Geometry check sheet. Reference: the model listing, model coordinates, mm. A direction names the side the tool comes from. Give positions to 0.01 mm unless a question says otherwise; leave off trailing zeros. Write each loop counter-clockwise with the first axis right and the second up, starting at its lowest first coordinate (ties: lowest second). Pieces come first, ordered by that corner, then holes. Notation, with made-up numbers: (76, 3) - (127, 3) arc R20 cw to (127, 7) - close; hole circle Ø11 at (57, 67). An arc over 180 degrees is marked (long way). Use a Markdown table: item, result.
```python
from build123d import *

# Parameters (mm, degrees)
SM_BASE_FLANGE_1_DEPTH = 171
SKETCH_5_OUTSIDE_W     = 426.43
SKETCH_5_OUTSIDE_H     = 439.1
SKETCH_5_OUTSIDE_R     = 515
CUT_EXTRUDE_2_DEPTH    = 250.150713085
FILLET_1_R             = 20
SKETCH_9_R             = 3.3
CUT_EXTRUDE_4_DEPTH    = 250.150713236


# Sheet-metal steps are written as plain solids
with BuildPart() as part:
    # Sketch 1 → Базовая кромка1 (new, symmetric)
    with BuildSketch(Plane.XY):
        with BuildLine():
            Line((150, 0), (-146.676192421, 0))
            ThreePointArc((-146.676192421, 0), (-160.818328044, -4.384471872), (-170, -16))
            Line((-170, -16), (-179.329523032, -12.4))
            ThreePointArc((-179.329523032, -12.4), (-166.475182294, 3.861739379), (-146.676192421, 10))
            Line((-146.676192421, 10), (150, 10))
            Line((150, 10), (150, 0))
        make_face()
    extrude(amount=SM_BASE_FLANGE_1_DEPTH, both=True)

    # Эскиз5 outside → Вырез-Вытянуть2 (cut, through all)
    with BuildSketch(Plane(origin=(0, 10, 0), x_dir=(1, 0, 0), z_dir=(0, 1, 0))):
        with Locations((-14.665, 0)):
            Rectangle(SKETCH_5_OUTSIDE_W, SKETCH_5_OUTSIDE_H)
        with Locations((-365, 0)):
            Circle(SKETCH_5_OUTSIDE_R, mode=Mode.SUBTRACT)
    extrude(amount=-CUT_EXTRUDE_2_DEPTH, mode=Mode.SUBTRACT)


with BuildPart() as cut_extrude_2_kept_piece:
    # of the separate pieces the step leaves, the one the design keeps (cut_extrude_2_pieces_kept)
    add(part.part.solids().sort_by_distance((-146.676192421, 10, -171))[0])

    # Скругление1
    fillet_1_edges = [cut_extrude_2_kept_piece.edges().sort_by_distance(p)[0] for p in [
        (-174.664761516, -14.2, -171),
        (-174.664761516, -14.2, 171),
    ]]
    fillet(fillet_1_edges, radius=FILLET_1_R)

    # Эскиз9 → Вырез-Вытянуть4 (cut, through all)
    with BuildSketch(Plane(origin=(0, 10, 0), x_dir=(1, 0, 0), z_dir=(0, 1, 0))):
        with Locations(Location((75.670476968, -155.5, 0), (0, 0, 180))):
            Circle(SKETCH_9_R)
        with Locations(Location((-84.329523032, -155.5, 0), (0, 0, 180))):
            Circle(SKETCH_9_R)
        with Locations((-84.329523032, 155.5)):
            Circle(SKETCH_9_R)
        with Locations((75.670476968, 155.5)):
            Circle(SKETCH_9_R)
    extrude(amount=-CUT_EXTRUDE_4_DEPTH, mode=Mode.SUBTRACT)


solid = cut_extrude_2_kept_piece.part
```
1) Set-up check for faces 1 (the cylindrical face through (-170.151, -9.829, 164.986)), 2 (the flat face through (4, 0, 2)): record each of +Z, -Z, +X, -X, +Y, -Y from which the full face is reachable in a straight line by a thin tool's end or side.
Working result:
| item | result |
|---|---|
| face 1 | +Z, -X, -Y |
| face 2 | +Z, -Z, +X, -Y |
2) Depth check by flat-ended pin: P1, Ø10, axis at x = -108.5, y = -7, coming from the +Z side; P2, Ø3, axis at x = -87, z = 43, coming from the -Y side; P3, Ø1, axis at y = -4, z = 20.5, coming from the +X side; P4, Ø1.5, axis at y = -9, z = -129.5, coming from the -X side. Enter the tip coordinate at first touch or a pass-through.
Working result:
| item | result |
|---|---|
| P1 | passes through |
| P2 | stops at y = 0 |
| P3 | stops at x = -159.43 |
| P4 | stops at x = -178.18 |
3) Material ranges on L1, parallel to X at y = 4.25, z = -155.5; L2, parallel to X at y = 5.25, z = 155.5; L3, parallel to Z at x = 77, y = 6.25, recorded low to high. Write a range as from..to.
Working result:
| item | result |
|---|---|
| L1 | x = -165.9..-87.63, -81.03..72.37, 78.97..125.96 |
| L2 | x = -164.28..-87.63, -81.03..72.37, 78.97..125.96 |
| L3 | z = -171..-158.52, -152.48..152.48, 158.52..171 |
4) Section check C-C on z = -145. Record the boundary of the cut face in (x, y), then the cut area to 3 significant figures.
Working result:
| item | result |
|---|---|
| outline | (-179.33, -12.4) - (-170, -16) arc R25 cw to (-146.68, 0) - (129.17, 0) - (129.17, 10) - (-146.68, 10) arc R35 ccw to start |
| area | 3,120 mm² |
5) Section check A-A on z = -3.5. Record the boundary of the cut face in (x, y).
Working result:
| item | result |
|---|---|
| outline | (-179.33, -12.4) - (-170, -16) arc R25 cw to (-146.68, 0) - (149.99, 0) - (149.99, 10) - (-146.68, 10) arc R35 ccw to start |
6) Section check B-B on x = -7.5. Record the boundary of the cut face in (y, z), then the cut area to 3 significant figures.
Working result:
| item | result |
|---|---|
| outline | (0, -171) - (10, -171) - (10, 171) - (0, 171) - close |
| area | 3,420 mm² |
